from build123d import *

# Parameters (mm, degrees)
F0_W     = 36
F0_H     = 36
F1_DEPTH = 5
F2_W     = 21
F2_H     = 21
F3_DEPTH = 15
F4_W     = 36
F4_H     = 36
F4_W_2   = 25
F4_H_2   = 25.4870138154
F5_DEPTH = 15
F6_R     = 2.5
F7_DEPTH = 40
F8_R     = 2.5
F9_DEPTH = 40


with BuildPart() as f1:
    # F0 (on Top) → F1 (new body)
    with BuildSketch(Plane.XY):
        Rectangle(F0_W, F0_H)
    extrude(amount=F1_DEPTH)

    # F2 (on face) → F3 (join)
    with BuildSketch(Plane.XY.offset(5)):
        Rectangle(F2_W, F2_H)
    extrude(amount=F3_DEPTH)

    # F4 (on face) → F5 (join)
    with BuildSketch(Plane.XY.offset(5)):
        Rectangle(F4_W, F4_H)
        Rectangle(F4_W_2, F4_H_2, mode=Mode.SUBTRACT)
    extrude(amount=F5_DEPTH)

    # F6 (on face) → F7 (cut)
    with BuildSketch(Plane.XZ.offset(18)):
        with Locations((0, 12.5)):
            Circle(F6_R)
    extrude(amount=-F7_DEPTH, mode=Mode.SUBTRACT)

    # F8 (on face) → F9 (cut)
    with BuildSketch(Plane(origin=(-18, 0, 0), x_dir=(0, -1, 0), z_dir=(-1, 0, 0))):
        with Locations((0, 12.5)):
            Circle(F8_R)
    extrude(amount=-F9_DEPTH, mode=Mode.SUBTRACT)


solid = f1.part
Input: part model. Units: mm. Frame: model coordinates. A direction names the side the tool comes from. Give positions to 0.01 mm unless a question says otherwise; leave off trailing zeros. Order: outer loops, then holes, each group sorted by start corner. A loop starts at its lowest first (then second) coordinate and runs counter-clockwise, first axis right, second up.
Q1. Section A-A on y = -10. Output: boundary loops of the cut face in (x, z).
Checked values:
outline: (-18, 0) - (18, 0) - (18, 20) - (12.5, 20) - (12.5, 5) - (10.5, 5) - (10.5, 20) - (-10.5, 20) - (-10.5, 5) - (-12.5, 5) - (-12.5, 20) - (-18, 20) - close; hole circle Ø5 at (0, 12.5)
Q2. Section C-C on z = 14. State how many separate pieces and enclosed holes the cut face has, and give its area (3 significant figures).
Checked values:
separate pieces: 8
enclosed holes: 0
area: 862 mm2
Q3. Contact query for a flat-ended pin moving along its axis: pin 1 Ø8 at (x, y) = (-6.5, -10) entering from -Z. Output: stop coordinate, or through.
Checked values:
pin 1: stops at z = 0
Q4. Set-up query: faces 4 (the flat face through (0, 0, 20)), 5 (the flat face through (-2.5, -10.5, 10.7)). Return all of +Z, -Z, +X, -X, +Y, -Y with unobstructed straight access to the full face (end or side cutting, diameter ignored); none if empty.
Checked values:
face 4: +Z, +X, -X, +Y, -Y
face 5: +Z
Q5. Section B-B on x = 15. Output: boundary loops of the cut face in (y, z).
Checked values:
outline: (-18, 0) - (18, 0) - (18, 20) - (-18, 20) - close; hole circle Ø5 at (0, 12.5)
Q6. Ray query, probe 1 along X at (y, z) = (-2, 19); probe 2 along X at (y, z) = (-3.25, 12.5); probe 3 along Z at (x, y) = (0, 14). Return the intervals inside material, ascending.
Checked values:
probe 1: x = -18 to -12.5, -10.5 to 10.5, 12.5 to 18
probe 2: x = -18 to -12.5, -10.5 to -2.5, 2.5 to 10.5, 12.5 to 18
probe 3: z = 0 to 10, 15 to 20
Q7. Draft query along Z for faces 1 (the flat face through (0, 0, 0)), 2 (the cylindrical face through (2.31, -6.49, 11.54)), 3 (the flat face through (-3, 12.744, 12)). Return one class per face: +Z half, -Z half, draft (parallel to the pull), parting line (faces both ways), or undercut.
Checked values:
face 1: -Z half
face 2: undercut
face 3: draft
